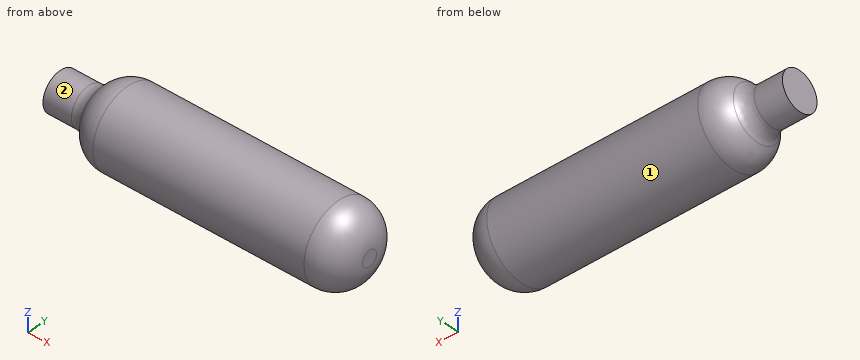
```python
from build123d import *

# Parameters (mm, degrees)
F0_R     = 3.175
F1_DEPTH = 6.35
F2_R     = 6.35
F3_DEPTH = 44.45
F4_R     = 5.08
F6_R     = 2.9585715778


# Not quite as in the source:
# - a fillet or chamfer that OpenCascade refuses, or shapes differently, is made with other operations: its cross-section is extruded or revolved along the edge and cut away or added


with BuildPart() as f1:
    # F0 (on Right) → F1 (new body)
    with BuildSketch(Plane.YZ):
        Circle(F0_R)
    extrude(amount=F1_DEPTH)

    # F2 (on face) → F3 (join)
    with BuildSketch(Plane.YZ.offset(6.35)):
        Circle(F2_R)
    extrude(amount=F3_DEPTH)

    # F4
    f4_edges = [f1.edges().sort_by_distance(p)[0] for p in [
        (50.8, -6.35, 0),
    ]]
    fillet(f4_edges, radius=F4_R)

    # F5: fillet of radius 5.08 on 1 edges, made by hand

    # F5_s1 → F5_t2 (revolve, cut)
    with BuildSketch(Plane.XY):
        with BuildLine():
            ThreePointArc((11.0592860393, 6.35), (8.2194797079, 5.4821134838), (6.35, 3.175))
            Line((6.35, 3.175), (6.35, 6.35))
            Line((6.35, 6.35), (11.0592860393, 6.35))
        make_face()
    revolve(axis=Axis((6.35, 0, 0), (1, 0, 0)), mode=Mode.SUBTRACT)

    # F6
    f6_edges = [f1.edges().sort_by_distance(p)[0] for p in [
        (6.35, -3.175, 0),
    ]]
    fillet(f6_edges, radius=F6_R)


solid = f1.part
```
Input: part model. Units: mm. Frame: model coordinates. Face numbers are marked on the shaded views. A direction names the side the tool comes from. Round coordinates to 2 decimals unless told otherwise and drop trailing zeros. Loops run counter-clockwise (first coordinate to the right, second up) from the corner with the lowest first, then second, coordinate; pieces in that order, holes last. Notation, with made-up numbers: (29, 21) -> (61, 21) arc R21 ccw to (61, 59) -> close; hole circle Ø10 at (73, 88). An arc over 180 degrees is marked (long way). Use one line per item in the form item = value. Start each with the question number.
Item 1: Set-up query: the marked faces 1 and 2. Return all of +Z, -Z, +X, -X, +Y, -Y with unobstructed straight access to the full face (end or side cutting, diameter ignored); none if empty.
Item 2: Contact query for flat-ended pins moving along their axis: pin 1 Ø2 at (x, y) = (40, 4) entering from -Z; pin 2 Ø1.5 at (x, y) = (39, 1) entering from +Z; pin 3 Ø2 at (x, z) = (18, -1.5) entering from +Y. Output: stop coordinate, or through.
Item 3: Material intervals for L1, parallel to Y at x = 17.5, z = -5.5; L2, parallel to Z at x = 32, y = 0.25; L3, parallel to X at y = 0, z = -5.25, sorted ascending. Write a range as from..to.
Item 4: Section query A-A on x = 23. Return the cut outline in (y, z), then the cut area to 3 significant figures.
Ans:
q1.face_1 = +X, -X
q1.face_2 = -X
q2.pin_1 = -5.6
q2.pin_2 = 6.35
q2.pin_3 = 6.33
q3.L1 = -3.17..3.17
q3.L2 = -6.35..6.35
q3.L3 = 7.9..48.88
q4.outline = circle Ø12.7 at (0, 0)
q4.area = 127 mm^2
